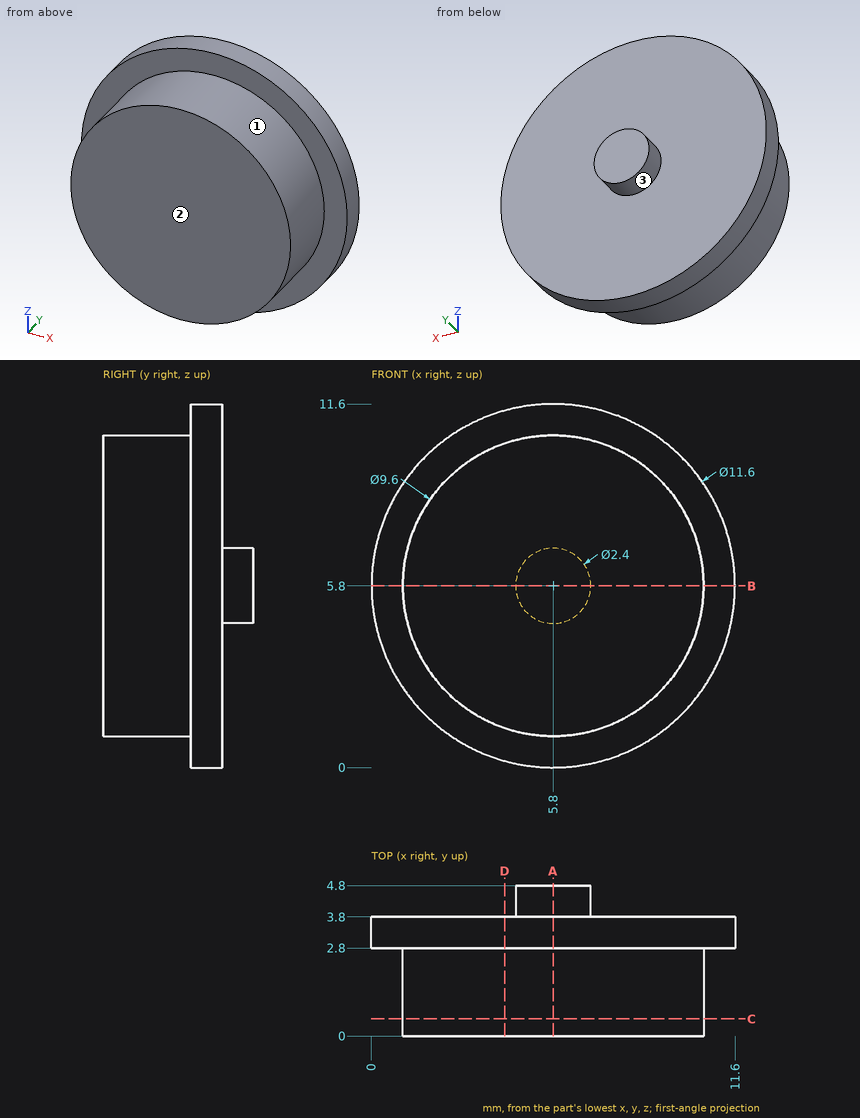
The figure shows three views and two pictorial views of one solid part (mm, origin at its lowest corner). Answer the questions. A direction names the side the tool comes from. Give positions to 0.01 mm unless a question says otherwise; leave off trailing zeros. Order: outer loops, then holes, each group sorted by start corner. A loop starts at its lowest first (then second) coordinate and runs counter-clockwise, first axis right, second up. Notation, with made-up numbers: M -27,4 L 25,4 A20 ccw 25,41 Z; hole C 31.25,48 d4. An arc over 180 degrees is marked long. Return JSON: item names as keys, results as strings.
Q1. Find section B-B, the plane z = 5.8. Write down the section's boundary in (x, y).
Answer below:
{"outline": "M 0,2.8 L 1,2.8 L 1,0 L 10.6,0 L 10.6,2.8 L 11.6,2.8 L 11.6,3.8 L 7,3.8 L 7,4.8 L 4.6,4.8 L 4.6,3.8 L 0,3.8 Z"}
Q2. Find section C-C, the plane y = 0.55. Write down the section's boundary in (x, z).
Answer below:
{"outline": "C 5.8,5.8 d9.6"}
Q3. Find section A-A, the plane x = 5.8. Write down the section's boundary in (y, z), and give its area (3 significant figures).
Answer below:
{"outline": "M 0,1 L 2.8,1 L 2.8,0 L 3.8,0 L 3.8,4.6 L 4.8,4.6 L 4.8,7 L 3.8,7 L 3.8,11.6 L 2.8,11.6 L 2.8,10.6 L 0,10.6 Z", "area": "40.9 mm^2"}
Q4. Which of the six approach directions +Z, -Z, +X, -X, +Y, -Y give full straight-line access (tool end or side, diameter ignored) to the marked faces 1, 2 and 3?
Answer below:
{"face 1": "-Y", "face 2": "+Z, -Z, +X, -X, -Y", "face 3": "+Y"}
Q5. Find the intervals of material crossed by line 1 along Y through (x, z) = (3.5, 3.75); line 2 along Y through (x, z) = (2.5, 1.5); line 3 along X through (y, z) = (0.8, 10), in increasing order. Write a range as [from, to].
Answer below:
{"line 1": "y = [0, 3.8]", "line 2": "y = [2.8, 3.8]", "line 3": "x = [3.48, 8.12]"}
Q6. This flat-tipped pin is pushed along its axis until it touches: pin 1 (1.5 mm diameter, centred on x = 3.5, z = 7, fed in from +Y). Where does it stop, or does it pass through?
Answer below:
{"pin 1": "stops at y = 3.8"}
Q7. Find section D-D, the plane x = 4.25. Write down the section's boundary in (y, z), and give its area (3 significant figures).
Answer below:
{"outline": "M 0,1.26 L 2.8,1.26 L 2.8,0.21 L 3.8,0.21 L 3.8,11.39 L 2.8,11.39 L 2.8,10.34 L 0,10.34 Z", "area": "36.6 mm^2"}
